Geometry check sheet. Reference: the model listing, model coordinates, mm. Give positions to 0.01 mm unless a question says otherwise; leave off trailing zeros. Write each loop counter-clockwise with the first axis right and the second up, starting at its lowest first coordinate (ties: lowest second). Pieces come first, ordered by that corner, then holes.
(1) Depth check by flat-ended pin: P1, Ø0.8, axis at y = 0, z = -44.5, coming from the -X side; P2, Ø4, axis at x = -27.5, z = 27.5, coming from the +Y side; P3, Ø0.8, axis at x = -49, y = 0, coming from the -Z side; P4, Ø0.5, axis at y = 0, z = -49, coming from the -X side. Enter the tip coordinate at first touch or a pass-through.
(2) Cross-section at A-A (x = 27.5). Record the boundary of the cut face in (y, z), and give its area (3 significant figures).
(3) Cross-section at D-D (z = 10.16). Record the boundary of the cut face in (x, y).
(4) Thickness scan on line 1 along Z through (x, y) = (6, 0.4); line 2 along Z through (x, y) = (29, -0.1); line 3 along Z through (x, y) = (43, 0.55). Record the ranges inside material, lowest first.
(5) Cross-section at C-C (x = -8.5). Record the boundary of the cut face in (y, z), and give its area (3 significant figures).
(6) Cross-section at B-B (z = 27.5). Record the boundary of the cut face in (x, y), and give its area (3 significant figures).
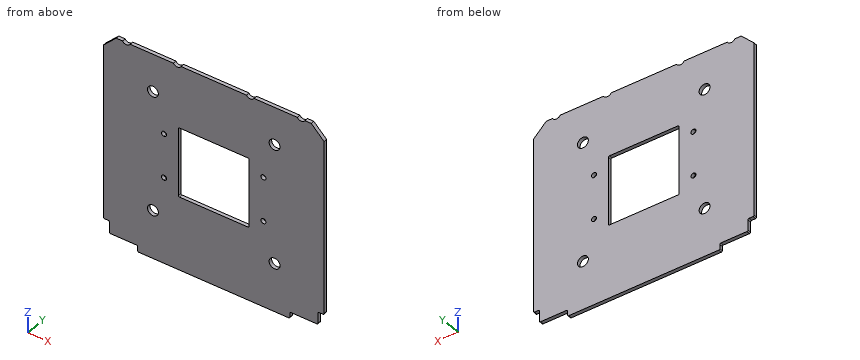
```python
from build123d import *

# Parameters (mm, degrees)
GENERICCARDPCBDEFINITION_START = -0.8
GENERICCARDPCBDEFINITION_DEPTH = 1.6
CUT_EXTRUDE1_REACH             = 72.517
CUT_EXTRUDE2_REACH             = 72.517
SKETCH8_R                      = 2.4575
FILLET1_R                      = 0.5


# Read off the part's stored shape, not the designer's step: GenericCardPCBDefinition
with BuildPart() as part:
    # GenericCardPCBDefinition outline → GenericCardPCBDefinition (new body)
    with BuildSketch(Plane(origin=(0, 0, 0), x_dir=(1, 0, 0), z_dir=(0, 1, 0)).offset(GENERICCARDPCBDEFINITION_START)):
        with BuildLine():
            Line((-49.9, -39), (-44.1, -44.8))
            Line((-44.1, -44.8), (-41.232050808, -44.8))
            ThreePointArc((-41.232050808, -44.8), (-39.5, -43.8), (-37.767949192, -44.8))
            Line((-37.767949192, -44.8), (-18.232050808, -44.8))
            ThreePointArc((-18.232050808, -44.8), (-16.5, -43.8), (-14.767949192, -44.8))
            Line((-14.767949192, -44.8), (14.767949192, -44.8))
            ThreePointArc((14.767949192, -44.8), (16.5, -43.8), (18.232050808, -44.8))
            Line((18.232050808, -44.8), (37.767949192, -44.8))
            ThreePointArc((37.767949192, -44.8), (39.5, -43.8), (41.232050808, -44.8))
            Line((41.232050808, -44.8), (44.1, -44.8))
            Line((44.1, -44.8), (49.9, -39))
            Line((49.9, -39), (49.9, 40.7))
            ThreePointArc((49.9, 40.7), (49.753553391, 41.053553391), (49.4, 41.2))
            Line((49.4, 41.2), (47.65, 41.2))
            ThreePointArc((47.65, 41.2), (47.296446609, 41.346446609), (47.15, 41.7))
            Line((47.15, 41.7), (47.15, 46.4))
            ThreePointArc((47.15, 46.4), (47.003553391, 46.753553391), (46.65, 46.9))
            Line((46.65, 46.9), (34.9, 46.9))
            ThreePointArc((34.9, 46.9), (34.546446609, 47.046446609), (34.4, 47.4))
            Line((34.4, 47.4), (34.4, 49.3))
            ThreePointArc((34.4, 49.3), (34.253553391, 49.653553391), (33.9, 49.8))
            Line((33.9, 49.8), (-33.9, 49.8))
            ThreePointArc((-33.9, 49.8), (-34.253553391, 49.653553391), (-34.4, 49.3))
            Line((-34.4, 49.3), (-34.4, 47.4))
            ThreePointArc((-34.4, 47.4), (-34.546446609, 47.046446609), (-34.9, 46.9))
            Line((-34.9, 46.9), (-46.65, 46.9))
            ThreePointArc((-46.65, 46.9), (-47.003553391, 46.753553391), (-47.15, 46.4))
            Line((-47.15, 46.4), (-47.15, 41.7))
            ThreePointArc((-47.15, 41.7), (-47.296446609, 41.346446609), (-47.65, 41.2))
            Line((-47.65, 41.2), (-49.4, 41.2))
            ThreePointArc((-49.4, 41.2), (-49.753553391, 41.053553391), (-49.9, 40.7))
            Line((-49.9, 40.7), (-49.9, -39))
        make_face()
    extrude(amount=GENERICCARDPCBDEFINITION_DEPTH)

    # Sketch7 → Cut-Extrude1 (cut, up to next)
    with BuildSketch(Plane(origin=(0, 0.8, 0), x_dir=(1, 0, 0), z_dir=(0, 1, 0)), mode=Mode.PRIVATE) as cut_extrude1_sk1:
        Polygon((16, 14.5), (16, -14.5), (16, -16), (-14.25, -16), (-14.5, -16), (-16, -16), (-16, -14.5), (-16, 14.5), (-16, 16), (-14.5, 16), (-14.25, 16), (2.7929, 16), (3.75, 16), (16, 16), align=None)
    cut_extrude1_tool1 = extrude(cut_extrude1_sk1.sketch, amount=-CUT_EXTRUDE1_REACH, mode=Mode.PRIVATE) & part.part
    add(cut_extrude1_tool1.solids().sort_by_distance((0, 0.8, 0))[0], mode=Mode.SUBTRACT)

    # Sketch8 → Cut-Extrude2 (cut, up to next)
    with BuildSketch(Plane(origin=(0, 0.8, 0), x_dir=(1, 0, 0), z_dir=(0, 1, 0)), mode=Mode.PRIVATE) as cut_extrude2_sk1:
        with Locations(Location((27.5, 27.5, 0), (0, 0, 270))):
            Circle(SKETCH8_R)
    cut_extrude2_tool1 = extrude(cut_extrude2_sk1.sketch, amount=-CUT_EXTRUDE2_REACH, mode=Mode.PRIVATE) & part.part
    # Sketch8 → Cut-Extrude2 (cut, up to next)
    with BuildSketch(Plane(origin=(0, 0.8, 0), x_dir=(1, 0, 0), z_dir=(0, 1, 0)), mode=Mode.PRIVATE) as cut_extrude2_sk2:
        with Locations(Location((-27.5, -27.5, 0), (0, 0, 270))):
            Circle(SKETCH8_R)
    cut_extrude2_tool2 = extrude(cut_extrude2_sk2.sketch, amount=-CUT_EXTRUDE2_REACH, mode=Mode.PRIVATE) & part.part
    # Sketch8 → Cut-Extrude2 (cut, up to next)
    with BuildSketch(Plane(origin=(0, 0.8, 0), x_dir=(1, 0, 0), z_dir=(0, 1, 0)), mode=Mode.PRIVATE) as cut_extrude2_sk3:
        with Locations(Location((27.5, -27.5, 0), (0, 0, 180))):
            Circle(SKETCH8_R)
    cut_extrude2_tool3 = extrude(cut_extrude2_sk3.sketch, amount=-CUT_EXTRUDE2_REACH, mode=Mode.PRIVATE) & part.part
    # Sketch8 → Cut-Extrude2 (cut, up to next)
    with BuildSketch(Plane(origin=(0, 0.8, 0), x_dir=(1, 0, 0), z_dir=(0, 1, 0)), mode=Mode.PRIVATE) as cut_extrude2_sk4:
        with Locations(Location((-27.5, 27.5, 0), (0, 0, 180))):
            Circle(SKETCH8_R)
    cut_extrude2_tool4 = extrude(cut_extrude2_sk4.sketch, amount=-CUT_EXTRUDE2_REACH, mode=Mode.PRIVATE) & part.part
    # Sketch8 → Cut-Extrude2 (cut, up to next)
    with BuildSketch(Plane(origin=(0, 0.8, 0), x_dir=(1, 0, 0), z_dir=(0, 1, 0)), mode=Mode.PRIVATE) as cut_extrude2_sk5:
        with BuildLine():
            ThreePointArc((-22.495277655, 11.290382806), (-23.6095, 10.16), (-22.495277655, 9.029617194))
            ThreePointArc((-22.495277655, 9.029617194), (-21.3485, 10.16), (-22.495277655, 11.290382806))
        make_face()
    cut_extrude2_tool5 = extrude(cut_extrude2_sk5.sketch, amount=-CUT_EXTRUDE2_REACH, mode=Mode.PRIVATE) & part.part
    # Sketch8 → Cut-Extrude2 (cut, up to next)
    with BuildSketch(Plane(origin=(0, 0.8, 0), x_dir=(1, 0, 0), z_dir=(0, 1, 0)), mode=Mode.PRIVATE) as cut_extrude2_sk6:
        with BuildLine():
            ThreePointArc((-22.504884895, -9.02979638), (-23.609238096, -10.135666951), (-22.553502979, -11.288042356))
            ThreePointArc((-22.553502979, -11.288042356), (-21.348761904, -10.184333049), (-22.504884895, -9.02979638))
        make_face()
    cut_extrude2_tool6 = extrude(cut_extrude2_sk6.sketch, amount=-CUT_EXTRUDE2_REACH, mode=Mode.PRIVATE) & part.part
    # Sketch8 → Cut-Extrude2 (cut, up to next)
    with BuildSketch(Plane(origin=(0, 0.8, 0), x_dir=(1, 0, 0), z_dir=(0, 1, 0)), mode=Mode.PRIVATE) as cut_extrude2_sk7:
        with BuildLine():
            ThreePointArc((22.479, 11.2905), (23.6095, 10.16), (22.479, 9.0295))
            ThreePointArc((22.479, 9.0295), (21.3485, 10.16), (22.479, 11.2905))
        make_face()
    cut_extrude2_tool7 = extrude(cut_extrude2_sk7.sketch, amount=-CUT_EXTRUDE2_REACH, mode=Mode.PRIVATE) & part.part
    # Sketch8 → Cut-Extrude2 (cut, up to next)
    with BuildSketch(Plane(origin=(0, 0.8, 0), x_dir=(1, 0, 0), z_dir=(0, 1, 0)), mode=Mode.PRIVATE) as cut_extrude2_sk8:
        with BuildLine():
            ThreePointArc((22.479, -9.0295), (23.6095, -10.16), (22.479, -11.2905))
            ThreePointArc((22.479, -11.2905), (21.3485, -10.16), (22.479, -9.0295))
        make_face()
    cut_extrude2_tool8 = extrude(cut_extrude2_sk8.sketch, amount=-CUT_EXTRUDE2_REACH, mode=Mode.PRIVATE) & part.part
    add(cut_extrude2_tool1.solids().sort_by_distance((27.5, 0.8, -27.5))[0], mode=Mode.SUBTRACT)
    add(cut_extrude2_tool2.solids().sort_by_distance((-27.5, 0.8, 27.5))[0], mode=Mode.SUBTRACT)
    add(cut_extrude2_tool3.solids().sort_by_distance((27.5, 0.8, 27.5))[0], mode=Mode.SUBTRACT)
    add(cut_extrude2_tool4.solids().sort_by_distance((-27.5, 0.8, -27.5))[0], mode=Mode.SUBTRACT)
    add(cut_extrude2_tool5.solids().sort_by_distance((-22.479, 0.8, -10.16))[0], mode=Mode.SUBTRACT)
    add(cut_extrude2_tool6.solids().sort_by_distance((-22.479, 0.8, 10.16))[0], mode=Mode.SUBTRACT)
    add(cut_extrude2_tool7.solids().sort_by_distance((22.479, 0.8, -10.16))[0], mode=Mode.SUBTRACT)
    add(cut_extrude2_tool8.solids().sort_by_distance((22.479, 0.8, 10.16))[0], mode=Mode.SUBTRACT)

    # Fillet1
    fillet1_edges = [part.edges().sort_by_distance(p)[0] for p in [
        (16, 0, -16),
        (16, 0, 16),
        (-16, 0, 16),
        (-16, 0, -16),
    ]]
    fillet(fillet1_edges, radius=FILLET1_R)


solid = part.part
```
Reply:
1. P1: stops at x = -47.15
1. P2: passes through
1. P3: stops at z = -41.2
1. P4: stops at x = -34.4
2. outline: (-0.8, -49.8) - (0.8, -49.8) - (0.8, -29.96) - (-0.8, -29.96) - close; (-0.8, -25.04) - (0.8, -25.04) - (0.8, 25.04) - (-0.8, 25.04) - close; (-0.8, 29.96) - (0.8, 29.96) - (0.8, 44.8) - (-0.8, 44.8) - close
2. area: 136 mm2
3. outline: (-49.9, -0.8) - (-23.61, -0.8) - (-23.61, 0.8) - (-49.9, 0.8) - close; (-21.35, -0.8) - (-16, -0.8) - (-16, 0.8) - (-21.35, 0.8) - close; (16, -0.8) - (21.35, -0.8) - (21.35, 0.8) - (16, 0.8) - close; (23.61, -0.8) - (49.9, -0.8) - (49.9, 0.8) - (23.61, 0.8) - close
4. line 1: z = -49.8 to -16, 16 to 44.8
4. line 2: z = -49.8 to -29.45, -25.55 to 25.55, 29.45 to 44.8
4. line 3: z = -46.9 to 44.8
5. outline: (-0.8, -49.8) - (0.8, -49.8) - (0.8, -16) - (-0.8, -16) - close; (-0.8, 16) - (0.8, 16) - (0.8, 44.8) - (-0.8, 44.8) - close
5. area: 100 mm2
6. outline: (-49.9, -0.8) - (-29.96, -0.8) - (-29.96, 0.8) - (-49.9, 0.8) - close; (-25.04, -0.8) - (25.04, -0.8) - (25.04, 0.8) - (-25.04, 0.8) - close; (29.96, -0.8) - (49.9, -0.8) - (49.9, 0.8) - (29.96, 0.8) - close
6. area: 144 mm2
